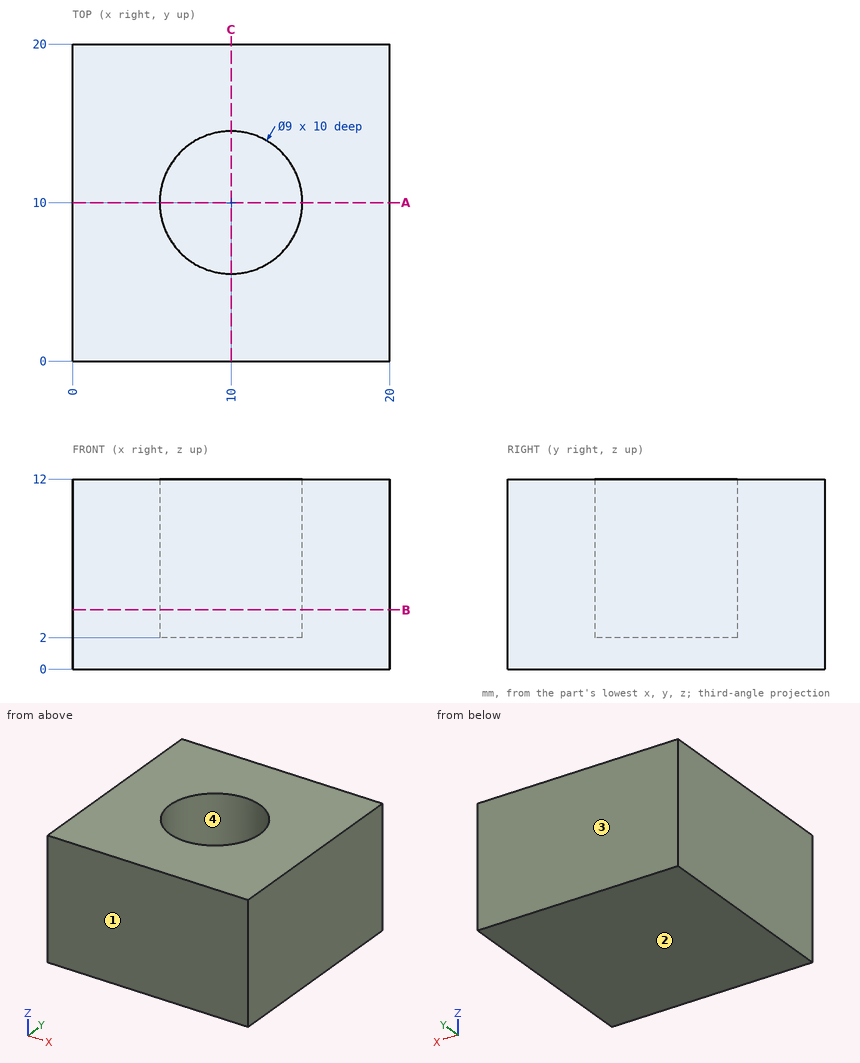
Study the drawing (mm; zero at the part's minimum x, y, z) and answer. Give positions to 0.01 mm unless a question says otherwise; leave off trailing zeros. Order: outer loops, then holes, each group sorted by start corner. A loop starts at its lowest first (then second) coordinate and runs counter-clockwise, first axis right, second up.
1. Each of these flat-tipped pins is pushed along its axis until it touches: P1, Ø8, axis at x = 10, y = 10, coming from the -Z side; P2, Ø4.5, axis at x = 9.5, y = 8, coming from the +Z side. Where does it stop, or does it pass through?
Result sheet:
P1: stops at z = 0
P2: stops at z = 2
2. Section A-A, the plane y = 10 is taken. Determine the outline of the cut face in (x, z).
Result sheet:
outline: (0, 0) - (20, 0) - (20, 12) - (14.5, 12) - (14.5, 2) - (5.5, 2) - (5.5, 12) - (0, 12) - close
3. The mould has two halves that part along Y. Classify the marked faces 1, 2, 3 and 4: released by +Y, released by -Y, zero draft, split by the parting line, or undercut.
Result sheet:
face 1: released by -Y
face 2: zero draft
face 3: released by +Y
face 4: undercut
4. Straight lines are drawn through the part: L1, parallel to Y at x = 10, z = 7.75; L2, parallel to Y at x = 11.25, z = 10.5; L3, parallel to Z at x = 10, y = 10.25. For each, find the intervals that lie inside material, in ascending order.
Result sheet:
L1: y = 0 to 5.5, 14.5 to 20
L2: y = 0 to 5.68, 14.32 to 20
L3: z = 0 to 2
5. Section B-B, the plane z = 3.75 is taken. Determine the outline of the cut face in (x, y), and give its area (3 significant figures).
Result sheet:
outline: (0, 0) - (20, 0) - (20, 20) - (0, 20) - close; hole circle Ø9 at (10, 10)
area: 336 mm2
